The listing builds one solid part. Answer for the finished solid, in the listing's coordinates (mm). A direction names the side the tool comes from. Give positions to 0.01 mm unless a question says otherwise; leave off trailing zeros. Order: outer loops, then holes, each group sorted by start corner. A loop starts at its lowest first (then second) coordinate and runs counter-clockwise, first axis right, second up. Notation, with made-up numbers: (39.5, 53.5) - (56.5, 53.5) arc R28 ccw to (56.5, 87.5) - close; hole circle Ø1 at (62, -32.5). An arc over 180 degrees is marked (long way). Use a Markdown table: item, result. Add a question column.
1) The mould has two halves that part along X. Classify faces 1 (the face through (-85, 34, 2)), 2 (the face through (67.488, 33.45, 134.36)), 3 (the face through (-1, 0, -2)): released by +X, released by -X, zero draft, split by the parting line, or undercut.
2) Find section B-B, the plane y = 34. Determine the outline of the cut face in (x, z).
3) For faces 4 (the face through (-1, 34, -124.5)), 5 (the face through (34.21, 25.55, 134.36)), determine the directions among +Z, -Z, +X, -X, +Y, -Y from which every point of the face is accessible in a straight line to the end or side of a thin tool.
4) Find section D-D, the plane y = 53. Determine the outline of the cut face in (x, z), plus the area to 3 significant figures.
5) Find section A-A, the plane x = 25. Determine the outline of the cut face in (y, z), plus the area to 3 significant figures.
6) Find section C-C, the plane x = -28. Determine the outline of the cut face in (y, z), plus the area to 3 significant figures.
7) Straight lines are drawn through the part: line 1 (Z direction, x = -5.5, y = 48.5); line 2 (Y direction, x = -61.5, z = 127.5). For each, find the intervals that lie inside material, in ascending order.
from build123d import *

# Parameters (mm, degrees)
SKETCH1_W           = 170
SKETCH1_H           = 249
BOSS_EXTRUDE1_DEPTH = 68
SKETCH2_R           = 12.5
BOSS_EXTRUDE2_DEPTH = 20


with BuildPart() as part:
    # Sketch1 → Boss-Extrude1 (new body)
    with BuildSketch(Plane(origin=(0, 0, 0), x_dir=(1, 0, 0), z_dir=(0, 1, 0))):
        Rectangle(SKETCH1_W, SKETCH1_H)
    extrude(amount=BOSS_EXTRUDE1_DEPTH)

    # Sketch2 → Boss-Extrude2 (add)
    with BuildSketch(Plane.XY.offset(124.5)):
        with Locations(Location((-65, 34, 0), (0, 0, 180))):
            Circle(SKETCH2_R)
        with Locations(Location((-35, 34, 0), (0, 0, 180))):
            Circle(SKETCH2_R)
        with Locations((-5, 34)):
            Circle(SKETCH2_R)
        with Locations(Location((25, 34, 0), (0, 0, 180))):
            Circle(SKETCH2_R)
        with Locations(Location((55, 34, 0), (0, 0, 180))):
            Circle(SKETCH2_R)
    extrude(amount=BOSS_EXTRUDE2_DEPTH)


solid = part.part
The answers:
| question | item | result |
|---|---|---|
| 1 | face 1 | released by -X |
| 1 | face 2 | undercut |
| 1 | face 3 | zero draft |
| 2 | outline | (-85, -124.5) - (85, -124.5) - (85, 124.5) - (67.5, 124.5) - (67.5, 144.5) - (42.5, 144.5) - (42.5, 124.5) - (37.5, 124.5) - (37.5, 144.5) - (12.5, 144.5) - (12.5, 124.5) - (7.5, 124.5) - (7.5, 144.5) - (-17.5, 144.5) - (-17.5, 124.5) - (-22.5, 124.5) - (-22.5, 144.5) - (-47.5, 144.5) - (-47.5, 124.5) - (-52.5, 124.5) - (-52.5, 144.5) - (-77.5, 144.5) - (-77.5, 124.5) - (-85, 124.5) - close |
| 3 | face 4 | -Z, +X, -X, +Y, -Y |
| 3 | face 5 | +Z |
| 4 | outline | (-85, -124.5) - (85, -124.5) - (85, 124.5) - (-85, 124.5) - close |
| 4 | area | 42,300 mm2 |
| 5 | outline | (0, -124.5) - (68, -124.5) - (68, 124.5) - (46.5, 124.5) - (46.5, 144.5) - (21.5, 144.5) - (21.5, 124.5) - (0, 124.5) - close |
| 5 | area | 17,400 mm2 |
| 6 | outline | (0, -124.5) - (68, -124.5) - (68, 124.5) - (44.36, 124.5) - (44.36, 144.5) - (23.64, 144.5) - (23.64, 124.5) - (0, 124.5) - close |
| 6 | area | 17,300 mm2 |
| 7 | line 1 | -124.5 to 124.5 |
| 7 | line 2 | 22 to 46 |
